Build history of the part. All positions in model axes, mm. Face numbers are marked on the shaded views. A direction names the side the tool comes from. Round coordinates to 2 decimals unless told otherwise and drop trailing zeros. Loops run counter-clockwise (first coordinate to the right, second up) from the corner with the lowest first, then second, coordinate; pieces in that order, holes last. Notation, with made-up numbers: M 11,71 L 56,71 A9 ccw 56,85 Z; hole C 51.25,-19 d3. An arc over 180 degrees is marked long. One line per item, written item: value.
Autodesk Inventor part; units mm, degrees
ref_plane "YZ Plane" through (0, 0, 0) normal (1, 0, 0) x (0, 1, 0)
ref_plane "XZ Plane" through (0, 0, 0) normal (0, 1, 0) x (-1, 0, 0)
ref_plane "XY Plane" through (0, 0, 0) normal (0, 0, 1) x (1, 0, 0)
sketch "Sketch1" plane through (0, 0, 0) normal (0, 1, 0) x (-1, 0, 0)
  circle A0 centre (0, 0) radius 2.5
  dimension "d0" = 5
extrude "Extrusion1" add sketch "Sketch1" along normal blind 30
ref_plane "Work Plane1" through (0, 3, 0) normal (0, -1, 0) x (1, 0, 0)
sketch "Sketch2" plane through (0, 3, 0) normal (0, -1, 0) x (1, 0, 0)
  circle A0 centre (0, 0) radius 6.5
  dimension "d4" = 13
extrude "Extrusion2" add sketch "Sketch2" against normal blind 25
properties part number "3D-roller"
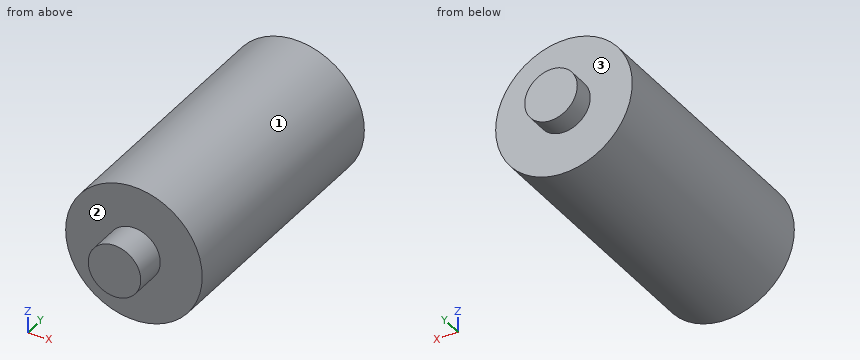
Item 1: Drop flat-ended pins along their axis: P1, Ø6, axis at y = 12.5, z = 4.5, coming from the -X side; P2, Ø4, axis at x = -5, y = 17, coming from the -Z side; P3, Ø2, axis at x = -3.5, y = 17, coming from the +Z side. Give the stop position or say it passes through.
Check values:
P1: stops at x = -6.32
P2: stops at z = -5.77
P3: stops at z = 6
Item 2: Slice it at A-A, the plane z = 0. Give the cut face in (x, y), and give its area (3 significant figures).
Check values:
outline: M -6.5,3 L -2.5,3 L -2.5,0 L 2.5,0 L 2.5,3 L 6.5,3 L 6.5,28 L 2.5,28 L 2.5,30 L -2.5,30 L -2.5,28 L -6.5,28 Z
area: 350 mm2
Item 3: Which spindle directions (+Z, -Z, +X, -X, +Y, -Y) get a long thin tool onto all of the face, cutting with end or side? Do the marked faces 1, 2 and 3. Say none if no direction does.
Check values:
face 1: +Y, -Y
face 2: -Y
face 3: +Y
Item 4: Slice it at C-C, the plane y = 24.25. Give the cut face in (x, z), and give its area (3 significant figures).
Check values:
outline: C 0,0 d13
area: 133 mm2
Item 5: Slice it at B-B, the plane x = 0. Give the cut face in (y, z).
Check values:
outline: M 0,-2.5 L 3,-2.5 L 3,-6.5 L 28,-6.5 L 28,-2.5 L 30,-2.5 L 30,2.5 L 28,2.5 L 28,6.5 L 3,6.5 L 3,2.5 L 0,2.5 Z
Item 6: Slice it at D-D, the plane x = 3.25. Give the cut face in (y, z).
Check values:
outline: M 3,-5.63 L 28,-5.63 L 28,5.63 L 3,5.63 Z
Item 7: Wall check: line 1 along Y through (x, z) = (1.5, 6); line 2 along Z through (x, y) = (-0.25, 6.75); line 3 along X through (y, z) = (8.25, 2.25). Give the ranges that are in metal, low to high.
Check values:
line 1: y = 3 to 28
line 2: z = -6.5 to 6.5
line 3: x = -6.1 to 6.1
